from build123d import *

# Parameters (mm, degrees)
MAIN_DEPTH                 = 20
ESQUISSE2_R                = 1.6
TOPHOLE_DEPTH              = 5
R_P_TITION_LIN_AIRE1_COUNT = 5
R_P_TITION_LIN_AIRE1_PITCH = 10


with BuildPart() as part:
    # Esquisse1 → Main (new body)
    with BuildSketch(Plane.XY):
        Polygon((-5, 0), (-5, 3), (-1.45, 3), (-1.45, 4), (1.45, 4), (1.45, 3), (5, 3), (5, 0), align=None)
    main = extrude(amount=MAIN_DEPTH)

    # Esquisse2 → TopHole (cut, through all)
    with BuildSketch(Plane(origin=(0, 4, 0), x_dir=(1, 0, 0), z_dir=(0, 1, 0))):
        with Locations((0, -5)):
            Circle(ESQUISSE2_R)
        with Locations((0, -15)):
            Circle(ESQUISSE2_R)
    tophole = extrude(amount=-TOPHOLE_DEPTH, mode=Mode.SUBTRACT)

    # Répétition linéaire1: Main, TopHole ×5
    with Locations(*[(-i * R_P_TITION_LIN_AIRE1_PITCH, 0, 0) for i in range(1, R_P_TITION_LIN_AIRE1_COUNT)]):
        add(main)
        add(tophole, mode=Mode.SUBTRACT)


solid = part.part
Work out the finished part from the listing and answer in its coordinate system (mm). A direction names the side the tool comes from. Round coordinates to 2 decimals unless told otherwise and drop trailing zeros. Order: outer loops, then holes, each group sorted by start corner. A loop starts at its lowest first (then second) coordinate and runs counter-clockwise, first axis right, second up. Notation, with made-up numbers: M 76.25,-16 L 90.25,-16 A22 ccw 90.25,15 Z; hole C 0.25,81 d3. An arc over 180 degrees is marked long. Put each result on its own line as item: value. Start each with the question number.
Q1. Flat-ended cylindrical pins translate along their axes: pin 1 (0.5 mm diameter, centred on y = 3.5, z = 2, fed in from -X); pin 2 (2 mm diameter, centred on x = -26.5, z = 12, fed in from +Y); pin 3 (1.1 mm diameter, centred on y = 3.5, z = 1.5, fed in from -X); pin 4 (0.8 mm diameter, centred on y = 3.5, z = 10.5, fed in from +X). Find the tip coordinate at first contact, or state that the pin passes through.
Q2. Section A-A, the plane z = 15 is taken. Write down the section's boundary in (x, y), and give its area (3 significant figures).
Q3. Section D-D, the plane z = 12.5 is taken. Write down the section's boundary in (x, y).
Q4. Section C-C, the plane y = 2.05 is taken. Give the number of separate pieces and of enclosed holes in the cut face, and give its area (3 significant figures).
Q5. For a pull along Z with two mould halves and no side action, classify faces 4 (the flat face through (1.45, 3.5, 2.1)), 5 (the cylindrical face through (-31.6, 2.03, 4.93)), 6 (the cylindrical face through (-41.6, 2.03, 4.93)) as pulls with the +Z half, pulls with the -Z half, needs draft (parallel to the pull), parting line crosses it, or undercut.
Q6. Straight lines are drawn through the part: L1, parallel to X at y = 3.6, z = 8.25; L2, parallel to X at y = 2.5, z = 15; L3, parallel to Z at x = -30, y = 2.8. For each, find the intervals that lie inside material, in ascending order. Write a range as [from, to].
Q7. A tool of negligible diameter and unlimited length cuts with its end or side. For faces 1 (the flat face through (-38.55, 3.5, 17.8)), 2 (the flat face through (-43, 3, 10)), 3 (the flat face through (3, 3, 10)), from which of +Z, -Z, +X, -X, +Y, -Y can it reach the whole face along a straight path? Write none if from no direction.
Q8. Section B-B, the plane x = -40 is taken. Write down the section's boundary in (y, z), and give its area (3 significant figures).
Findings below:
1. pin 1: stops at x = -41.45
1. pin 2: stops at y = 3
1. pin 3: stops at x = -45
1. pin 4: stops at x = 1.45
2. outline: M -45,0 L -41.6,0 L -41.6,3 L -45,3 Z; M -38.4,0 L -31.6,0 L -31.6,3 L -38.4,3 Z; M -28.4,0 L -21.6,0 L -21.6,3 L -28.4,3 Z; M -18.4,0 L -11.6,0 L -11.6,3 L -18.4,3 Z; M -8.4,0 L -1.6,0 L -1.6,3 L -8.4,3 Z; M 1.6,0 L 5,0 L 5,3 L 1.6,3 Z
2. area: 102 mm^2
3. outline: M -45,0 L 5,0 L 5,3 L 1.45,3 L 1.45,4 L -1.45,4 L -1.45,3 L -8.55,3 L -8.55,4 L -11.45,4 L -11.45,3 L -18.55,3 L -18.55,4 L -21.45,4 L -21.45,3 L -28.55,3 L -28.55,4 L -31.45,4 L -31.45,3 L -38.55,3 L -38.55,4 L -41.45,4 L -41.45,3 L -45,3 Z
4. separate pieces: 1
4. enclosed holes: 10
4. area: 920 mm^2
5. face 4: needs draft
5. face 5: undercut
5. face 6: undercut
6. L1: x = [-41.45, -38.55], [-31.45, -28.55], [-21.45, -18.55], [-11.45, -8.55], [-1.45, 1.45]
6. L2: x = [-45, -41.6], [-38.4, -31.6], [-28.4, -21.6], [-18.4, -11.6], [-8.4, -1.6], [1.6, 5]
6. L3: z = [0, 3.4], [6.6, 13.4], [16.6, 20]
7. face 1: +Z, -Z, +Y
7. face 2: +Z, -Z, -X, +Y
7. face 3: +Z, -Z, +X, +Y
8. outline: M 0,0 L 4,0 L 4,3.4 L 0,3.4 Z; M 0,6.6 L 4,6.6 L 4,13.4 L 0,13.4 Z; M 0,16.6 L 4,16.6 L 4,20 L 0,20 Z
8. area: 54.4 mm^2
